from build123d import *

# Parameters (mm, degrees)
PAD012_DEPTH            = 6
FILLET002_R             = 2
FILLET003_R             = 2
BODY011_PLACEMENT_ANGLE = 180


with BuildPart() as part:
    # Sketch025 → Pad012 (new body)
    with BuildSketch(Plane.YZ):
        with BuildLine():
            Line((6.011752, 0), (36.011752, 0))
            Line((36.011752, 0), (36.011752, -2))
            ThreePointArc((36.011752, -2), (17.671346, -11.659594), (8.011752, -30))
            Line((8.011752, -30), (6.011752, -30))
            Line((6.011752, -30), (6.011752, 0))
        make_face()
    extrude(amount=PAD012_DEPTH)

    # Fillet002
    fillet002_edges = [part.edges().sort_by_distance(p)[0] for p in [
        (3, 36.011752, -2),
    ]]
    fillet(fillet002_edges, radius=FILLET002_R)

    # Fillet003
    fillet003_edges = [part.edges().sort_by_distance(p)[0] for p in [
        (3, 8.011752, -30),
    ]]
    fillet(fillet003_edges, radius=FILLET003_R)


with BuildPart() as part_1:
    # Body011 placement: moved
    add(part.part.moved(Location((2, 0, 8))).rotate(Axis((2, 0, 8), (0, 1, 0)), BODY011_PLACEMENT_ANGLE))


solid = part_1.part
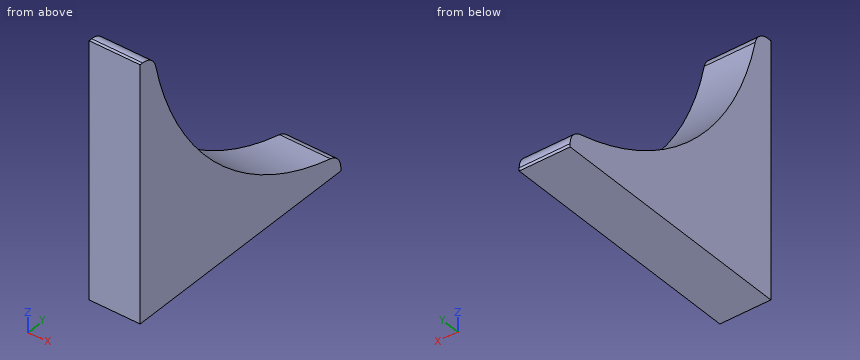
Geometry check sheet. Reference: the model listing, model coordinates, mm. Round coordinates to 2 decimals unless told otherwise and drop trailing zeros. Write each loop counter-clockwise with the first axis right and the second up, starting at its lowest first coordinate (ties: lowest second). Pieces come first, ordered by that corner, then holes. Notation, with made-up numbers: (89, 49.25) - (97, 49.25) arc R16 cw to (97, 57.25) - close; hole circle Ø11 at (-28, 74). An arc over 180 degrees is marked (long way). One line per item, written item: value.
1. Cross-section at A-A on x = 0.75. Record the boundary of the cut face in (y, z), and give its area (3 significant figures).
The answers:
outline: (6.01, 8) - (36.01, 8) - (36.01, 8.38) arc R2 ccw to (34.47, 10.32) arc R35 cw to (8.34, 36.45) arc R2 ccw to (6.39, 38) - (6.01, 38) - close
area: 342 mm^2
2. Cross-section at B-B on z = 24. Record the boundary of the cut face in (x, y), and give its area (3 significant figures).
The answers:
outline: (-4, 6.01) - (2, 6.01) - (2, 13.99) - (-4, 13.99) - close
area: 47.8 mm^2
3. Depth check by flat-ended pin: pin 1 Ø12 at (y, z) = (13.5, 28.5) entering from -X. Enter the tip coordinate at first touch or a pass-through.
The answers:
pin 1: stops at x = -4
4. Scan lines: L1, parallel to Z at x = -1, y = 12.5; L2, parallel to Y at x = -1.25, z = 31.5; L3, parallel to Y at x = -1.5, z = 33. Record each from-to range of solid material in increasing order.
The answers:
L1: z = 8 to 26.25
L2: y = 6.01 to 9.89
L3: y = 6.01 to 9.33
5. Cross-section at C-C on y = 19.25. Record the boundary of the cut face in (x, z).
The answers:
outline: (-4, 8) - (2, 8) - (2, 18.18) - (-4, 18.18) - close
